Model file for the job. Use its own axes, mm. A direction names the side the tool comes from. Round coordinates to 2 decimals unless told otherwise and drop trailing zeros. Order: outer loops, then holes, each group sorted by start corner. A loop starts at its lowest first (then second) coordinate and runs counter-clockwise, first axis right, second up. Notation, with made-up numbers: (-22.75, -39) - (2.25, -39) arc R31 ccw to (2.25, -13) - close; hole circle Ø11 at (-31.5, -22.5). An arc over 180 degrees is marked (long way). Put each result on its own line as item: value. Start each with the question number.
Item 1: Saw through at A-A on z = 49. List the corners of the cut face in (x, y), plus the area to 3 significant figures.
Item 2: Mould opens along X. For faces 5 (the face through (129, -3, 0)), 6 (the face through (4, -1, 44)) say: pulls with the +X half, pulls with the -X half, needs draft (parallel to the pull), parting line crosses it, or undercut.
Item 3: Which spindle directions (+Z, -Z, +X, -X, +Y, -Y) get a long thin tool onto all of the face, cutting with end or side? Do faces 1 (the face through (136, -2.25, 43)), 2 (the face through (133, -3.75, 43)), 3 (the face through (5, -5, 44)), 4 (the face through (4, -6, 43)). Say none if no direction does.
Item 4: Saw through at B-B on x = 242. List the corners of the cut face in (y, z).
Item 5: Probe probe 1 along X at (y, z) = (-2.5, 51); probe 2 along Y at (x, z) = (210.5, 56); probe 3 along X at (y, z) = (-1.85, 52). List the from-to ranges inside material, lowest first.
Item 6: Pin check, flat tips, straight feed: pin 1 Ø12 at (x, z) = (183.5, 75.5) entering from +Y; pin 2 Ø2 at (y, z) = (-3, 59) entering from -X; pin 3 Ø2 at (x, y) = (39, -1) entering from +Z; pin 4 Ø1.5 at (x, z) = (89.5, 46) entering from -Y. Stop position of each tip, or through.
```python
from build123d import *

# Parameters (mm, degrees)
EXTRUDE_1_DEPTH     = 87
CUT_EXTRUDE_1_DEPTH = 274.287394514


with BuildPart() as part:
    # 草图1 → 凸台-拉伸1 (new body)
    with BuildSketch(Plane.XY):
        with BuildLine():
            Line((9, -1.25), (9, -1))
            ThreePointArc((9, -1), (8.707106781, -0.292893219), (8, 0))
            Line((8, 0), (1, 0))
            ThreePointArc((1, 0), (0.292893219, -0.292893219), (0, -1))
            Line((0, -1), (0, -5))
            ThreePointArc((0, -5), (0.292893219, -5.707106781), (1, -6))
            Line((1, -6), (8, -6))
            ThreePointArc((8, -6), (8.707106781, -5.707106781), (9, -5))
            Line((9, -5), (9, -4.75))
            ThreePointArc((9, -4.75), (9.292893219, -4.042893219), (10, -3.75))
            Line((10, -3.75), (259, -3.75))
            Line((259, -3.75), (259, -2.25))
            Line((259, -2.25), (10, -2.25))
            ThreePointArc((10, -2.25), (9.292893219, -1.957106781), (9, -1.25))
        make_face()
    extrude(amount=EXTRUDE_1_DEPTH)

    # 草图2 → 切除-拉伸1 (cut, through all)
    with BuildSketch(Plane.XY.offset(87)):
        with BuildLine():
            Line((2, -1), (7, -1))
            ThreePointArc((7, -1), (7.707106781, -1.292893219), (8, -2))
            Line((8, -2), (8, -4))
            ThreePointArc((8, -4), (7.707106781, -4.707106781), (7, -5))
            Line((7, -5), (2, -5))
            ThreePointArc((2, -5), (1.292893219, -4.707106781), (1, -4))
            Line((1, -4), (1, -2))
            ThreePointArc((1, -2), (1.292893219, -1.292893219), (2, -1))
        make_face()
    extrude(amount=-CUT_EXTRUDE_1_DEPTH, mode=Mode.SUBTRACT)


solid = part.part
```
Results found:
1. outline: (0, -5) arc R1 ccw to (1, -6) - (8, -6) arc R1 ccw to (9, -5) - (9, -4.75) arc R1 cw to (10, -3.75) - (259, -3.75) - (259, -2.25) - (10, -2.25) arc R1 cw to (9, -1.25) - (9, -1) arc R1 ccw to (8, 0) - (1, 0) arc R1 ccw to (0, -1) - close; hole (1, -4) arc R1 ccw to (2, -5) - (7, -5) arc R1 ccw to (8, -4) - (8, -2) arc R1 ccw to (7, -1) - (2, -1) arc R1 ccw to (1, -2) - close
1. area: 401 mm²
2. face 5: needs draft
2. face 6: undercut
3. face 1: +Z, -Z, +X, +Y
3. face 2: +Z, -Z, +X, -Y
3. face 3: +Z, -Z
3. face 4: +Z, -Z, +X, -X, -Y
4. outline: (-3.75, 0) - (-2.25, 0) - (-2.25, 87) - (-3.75, 87) - close
5. probe 1: x = 0 to 1, 8 to 259
5. probe 2: y = -3.75 to -2.25
5. probe 3: x = 0 to 1.01, 7.99 to 9.2
6. pin 1: stops at y = -2.25
6. pin 2: stops at x = 0
6. pin 3: passes through
6. pin 4: stops at y = -3.75
